```python
from build123d import *

# Parameters (mm, degrees)
SKETCH_1_R      = 2.55
EXTRUDE_1_DEPTH = 1.1
SKETCH_2_R      = 2.55
SKETCH_2_R_2    = 1.5
EXTRUDE_2_DEPTH = 0.9


with BuildPart() as part:
    # Эскиз1 → Бобышка-Вытянуть1 (new body)
    with BuildSketch(Plane(origin=(0, 0, 0), x_dir=(1, 0, 0), z_dir=(0, 1, 0))):
        with BuildLine():
            Line((33.15, -24), (-33.15, -24))
            ThreePointArc((-33.15, -24), (-34.210660172, -23.560660172), (-34.65, -22.5))
            Line((-34.65, -22.5), (-34.65, 22.5))
            ThreePointArc((-34.65, 22.5), (-34.210660172, 23.560660172), (-33.15, 24))
            Line((-33.15, 24), (33.15, 24))
            ThreePointArc((33.15, 24), (34.210660172, 23.560660172), (34.65, 22.5))
            Line((34.65, 22.5), (34.65, -22.5))
            ThreePointArc((34.65, -22.5), (34.210660172, -23.560660172), (33.15, -24))
        make_face()
        with Locations(Location((-31.5, 21, 0), (0, 0, 270))):
            Circle(SKETCH_1_R, mode=Mode.SUBTRACT)
        with Locations(Location((31.5, 21, 0), (0, 0, 270))):
            Circle(SKETCH_1_R, mode=Mode.SUBTRACT)
        with Locations(Location((31.5, -21, 0), (0, 0, 270))):
            Circle(SKETCH_1_R, mode=Mode.SUBTRACT)
        with Locations(Location((-31.5, -21, 0), (0, 0, 270))):
            Circle(SKETCH_1_R, mode=Mode.SUBTRACT)
    extrude(amount=EXTRUDE_1_DEPTH)

    # Эскиз2 → Бобышка-Вытянуть2 (add)
    # profile 1 of 4: a face of its own
    with BuildSketch(Plane(origin=(0, 0.1, 0), x_dir=(-1, 0, 0), z_dir=(0, -1, 0))):
        with Locations(Location((31.5, -21, 0), (0, 0, 90))):
            Circle(SKETCH_2_R)
        with Locations(Location((31.5, -21, 0), (0, 0, 90))):
            Circle(SKETCH_2_R_2, mode=Mode.SUBTRACT)
    # profile 2 of 4: a face of its own
    with BuildSketch(Plane(origin=(0, 0.1, 0), x_dir=(-1, 0, 0), z_dir=(0, -1, 0))):
        with Locations(Location((-31.5, -21, 0), (0, 0, 90))):
            Circle(SKETCH_2_R)
        with Locations(Location((-31.5, -21, 0), (0, 0, 90))):
            Circle(SKETCH_2_R_2, mode=Mode.SUBTRACT)
    # profile 3 of 4: a face of its own
    with BuildSketch(Plane(origin=(0, 0.1, 0), x_dir=(-1, 0, 0), z_dir=(0, -1, 0))):
        with Locations(Location((-31.5, 21, 0), (0, 0, 90))):
            Circle(SKETCH_2_R)
        with Locations(Location((-31.5, 21, 0), (0, 0, 90))):
            Circle(SKETCH_2_R_2, mode=Mode.SUBTRACT)
    # profile 4 of 4: a face of its own
    with BuildSketch(Plane(origin=(0, 0.1, 0), x_dir=(-1, 0, 0), z_dir=(0, -1, 0))):
        with Locations(Location((31.5, 21, 0), (0, 0, 90))):
            Circle(SKETCH_2_R)
        with Locations(Location((31.5, 21, 0), (0, 0, 90))):
            Circle(SKETCH_2_R_2, mode=Mode.SUBTRACT)
    extrude(amount=-EXTRUDE_2_DEPTH)


solid = part.part
```
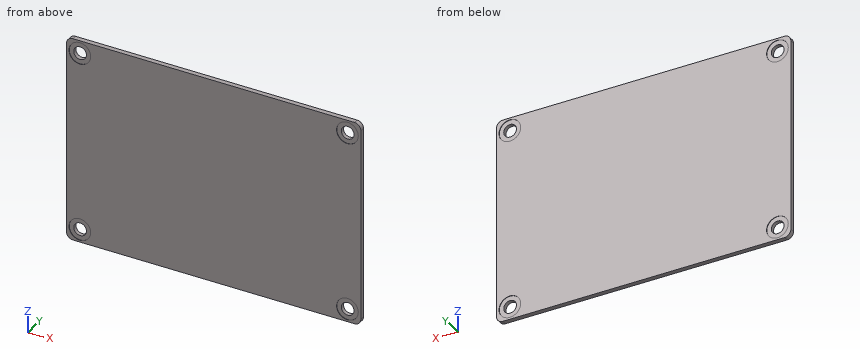
The model under review builds one solid part; all positions refer to its coordinate system, in mm. Round coordinates to 2 decimals unless told otherwise and drop trailing zeros. Loops run counter-clockwise (first coordinate to the right, second up) from the corner with the lowest first, then second, coordinate; pieces in that order, holes last. Notation, with made-up numbers: M 61,33.25 L 95,33.25 A26 cw 95,51.25 Z; hole C 0.25,41 d2. An arc over 180 degrees is marked long. Write item = value, one per line.
Item 1: Take a section at B-B on x = -31.5. Write out the cut boundary in (y, z).
Return value:
outline = M 0,-24 L 1.1,-24 L 1.1,-23.55 L 1,-23.55 L 1,-22.5 L 0.1,-22.5 L 0.1,-23.55 L 0,-23.55 Z; M 0,-18.45 L 0.1,-18.45 L 0.1,-19.5 L 1,-19.5 L 1,-18.45 L 1.1,-18.45 L 1.1,18.45 L 1,18.45 L 1,19.5 L 0.1,19.5 L 0.1,18.45 L 0,18.45 Z; M 0,23.55 L 0.1,23.55 L 0.1,22.5 L 1,22.5 L 1,23.55 L 1.1,23.55 L 1.1,24 L 0,24 Z
Item 2: Take a section at A-A on z = -21. Write out the cut boundary in (x, y), then the cut area to 3 significant figures.
Return value:
outline = M -34.65,0 L -34.05,0 L -34.05,0.1 L -33,0.1 L -33,1 L -34.05,1 L -34.05,1.1 L -34.65,1.1 Z; M -30,0.1 L -28.95,0.1 L -28.95,0 L 28.95,0 L 28.95,0.1 L 30,0.1 L 30,1 L 28.95,1 L 28.95,1.1 L -28.95,1.1 L -28.95,1 L -30,1 Z; M 33,0.1 L 34.05,0.1 L 34.05,0 L 34.65,0 L 34.65,1.1 L 34.05,1.1 L 34.05,1 L 33,1 Z
area = 68.8 mm2
Item 3: Insertion check: P1, Ø1.5, axis at x = 31.5, z = -22, coming from the -Y side. The pin has a flat end and moves straight along its axis. Give the tip position at first contact, or say it passes through.
Return value:
P1 = 0.1
Item 4: For line 1 (X direction, y = 0.05, z = -21); line 2 (X direction, y = 0.6, z = -21), list the stretches that pass through material, from the lowest coordinate up. Write a range as [from, to].
Return value:
line_1 = [-34.65, -34.05], [-28.95, 28.95], [34.05, 34.65]
line_2 = [-34.65, -33], [-30, 30], [33, 34.65]
